```python
from build123d import *

# Parameters (mm, degrees)
F0_R     = 60
F1_DEPTH = 5
F3_DEPTH = 5.001
F4_R     = 58
F5_DEPTH = 3


with BuildPart() as f1:
    # F0 (on Top) → F1 (new body)
    with BuildSketch(Plane.XY):
        Circle(F0_R)
    extrude(amount=F1_DEPTH)

    # F2 (on face) → F3 (cut, through all)
    with BuildSketch(Plane.XY.offset(5)):
        with BuildLine():
            Line((-2.741307, 50.860289), (-2.800394, 53.905666))
            ThreePointArc((-2.800394, 53.905666), (-26.810197, 46.78331), (-44.999208, 29.568246))
            Line((-44.999208, 29.568246), (-42.39098, 27.998535))
            ThreePointArc((-42.39098, 27.998535), (-39.422273, 32.097611), (-36.032442, 35.855893))
            Line((-36.032442, 35.855893), (-31.764433, 31.624433))
            ThreePointArc((-31.764433, 31.624433), (-22.28061, 38.940283), (-11.190111, 43.46415))
            Line((-11.190111, 43.46415), (-12.704825, 49.321402))
            ThreePointArc((-12.704825, 49.321402), (-7.767263, 50.377001), (-2.741307, 50.860289))
        make_face()
        with BuildLine():
            Line((-53.808689, 0), (-44.738998, 0))
            ThreePointArc((-44.738998, 0), (-44.333174, 5.994104), (-43.11711, 11.877569))
            Line((-43.11711, 11.877569), (-48.95667, 13.487858))
            ThreePointArc((-48.95667, 13.487858), (-47.364057, 18.296418), (-45.259964, 22.904178))
            Line((-45.259964, 22.904178), (-47.967557, 24.430441))
            ThreePointArc((-47.967557, 24.430441), (-52.328709, 12.559654), (-53.808689, 0))
        make_face()
        with BuildLine():
            ThreePointArc((-43.11711, -11.832559), (-44.330124, -5.971391), (-44.738998, 0))
            Line((-44.738998, 0), (-53.808689, 0))
            ThreePointArc((-53.808689, 0), (-52.334607, -12.524554), (-47.995206, -24.365457))
            Line((-47.995206, -24.365457), (-45.342475, -22.814272))
            ThreePointArc((-45.342475, -22.814272), (-47.380636, -18.21008), (-48.948068, -13.42512))
            Line((-48.948068, -13.42512), (-43.11711, -11.832559))
        make_face()
        with BuildLine():
            Line((-42.377204, -28.020563), (-45.023724, -29.548192))
            ThreePointArc((-45.023724, -29.548192), (-26.781507, -46.767749), (-2.742129, -53.937126))
            Line((-2.742129, -53.937126), (-2.742129, -50.906584))
            ThreePointArc((-2.742129, -50.906584), (-7.777308, -50.376699), (-12.725699, -49.305607))
            Line((-12.725699, -49.305607), (-11.188747, -43.482557))
            ThreePointArc((-11.188747, -43.482557), (-22.268417, -38.947418), (-31.75433, -31.643718))
            Line((-31.75433, -31.643718), (-36.039297, -35.877891))
            ThreePointArc((-36.039297, -35.877891), (-39.414393, -32.115507), (-42.377204, -28.020563))
        make_face()
        with BuildLine():
            Line((0, -36.08707), (0, 0))
            Line((0, 0), (-17.828856, 0))
            ThreePointArc((-17.828856, 0), (-17.551636, -3.026807), (-16.733946, -5.954228))
            Line((-16.733946, -5.954228), (-33.773992, -11.896965))
            ThreePointArc((-33.773992, -11.896965), (-30.963522, -18.016735), (-27.060224, -23.504412))
            Line((-27.060224, -23.504412), (-13.459581, -11.657408))
            ThreePointArc((-13.459581, -11.657408), (-8.750525, -15.531259), (-3.038921, -17.66656))
            Line((-3.038921, -17.66656), (-6.482814, -35.405271))
            ThreePointArc((-6.482814, -35.405271), (-3.256267, -35.887467), (0, -36.08707))
        make_face()
        with BuildLine():
            Line((17.828856, 0), (0, 0))
            Line((0, 0), (0, -36.08707))
            ThreePointArc((0, -36.08707), (3.256267, -35.887467), (6.482814, -35.405271))
            Line((6.482814, -35.405271), (3.038921, -17.66656))
            ThreePointArc((3.038921, -17.66656), (8.750525, -15.531259), (13.459581, -11.657408))
            Line((13.459581, -11.657408), (27.060224, -23.504412))
            ThreePointArc((27.060224, -23.504412), (30.963522, -18.016735), (33.773992, -11.896965))
            Line((33.773992, -11.896965), (16.733946, -5.954228))
            ThreePointArc((16.733946, -5.954228), (17.551636, -3.026807), (17.828856, 0))
        make_face()
        with BuildLine():
            Line((0, 36.015704), (0, 0))
            Line((0, 0), (17.828856, 0))
            ThreePointArc((17.828856, 0), (17.554095, 3.040658), (16.733946, 5.981483))
            Line((16.733946, 5.981483), (33.78848, 11.882508))
            ThreePointArc((33.78848, 11.882508), (30.964356, 18.004289), (27.054407, 23.496481))
            Line((27.054407, 23.496481), (13.461306, 11.712858))
            ThreePointArc((13.461306, 11.712858), (8.780542, 15.595833), (3.079093, 17.712558))
            Line((3.079093, 17.712558), (6.480865, 35.418753))
            ThreePointArc((6.480865, 35.418753), (3.252606, 35.849388), (0, 36.015704))
        make_face()
        with BuildLine():
            Line((-17.828856, 0), (0, 0))
            Line((0, 0), (0, 36.015704))
            ThreePointArc((0, 36.015704), (-3.252606, 35.849388), (-6.480865, 35.418753))
            Line((-6.480865, 35.418753), (-3.079093, 17.712558))
            ThreePointArc((-3.079093, 17.712558), (-8.780542, 15.595833), (-13.461306, 11.712858))
            Line((-13.461306, 11.712858), (-27.054407, 23.496481))
            ThreePointArc((-27.054407, 23.496481), (-30.964356, 18.004289), (-33.78848, 11.882508))
            Line((-33.78848, 11.882508), (-16.733946, 5.981483))
            ThreePointArc((-16.733946, 5.981483), (-17.554095, 3.040658), (-17.828856, 0))
        make_face()
        with BuildLine():
            Line((2.742129, -50.906584), (2.742129, -53.937126))
            ThreePointArc((2.742129, -53.937126), (26.781507, -46.767749), (45.023724, -29.548192))
            Line((45.023724, -29.548192), (42.377204, -28.020563))
            ThreePointArc((42.377204, -28.020563), (39.414393, -32.115507), (36.039297, -35.877891))
            Line((36.039297, -35.877891), (31.75433, -31.643718))
            ThreePointArc((31.75433, -31.643718), (22.268417, -38.947418), (11.188747, -43.482557))
            Line((11.188747, -43.482557), (12.725699, -49.305607))
            ThreePointArc((12.725699, -49.305607), (7.777308, -50.376699), (2.742129, -50.906584))
        make_face()
        with BuildLine():
            ThreePointArc((43.11711, 11.877569), (44.333174, 5.994104), (44.738998, 0))
            Line((44.738998, 0), (53.808689, 0))
            ThreePointArc((53.808689, 0), (52.328709, 12.559654), (47.967557, 24.430441))
            Line((47.967557, 24.430441), (45.259964, 22.904178))
            ThreePointArc((45.259964, 22.904178), (47.364057, 18.296418), (48.95667, 13.487858))
            Line((48.95667, 13.487858), (43.11711, 11.877569))
        make_face()
        with BuildLine():
            Line((53.808689, 0), (44.738998, 0))
            ThreePointArc((44.738998, 0), (44.330124, -5.971391), (43.11711, -11.832559))
            Line((43.11711, -11.832559), (48.948068, -13.42512))
            ThreePointArc((48.948068, -13.42512), (47.380636, -18.21008), (45.342475, -22.814272))
            Line((45.342475, -22.814272), (47.995206, -24.365457))
            ThreePointArc((47.995206, -24.365457), (52.334607, -12.524554), (53.808689, 0))
        make_face()
        with BuildLine():
            Line((42.39098, 27.998535), (44.999208, 29.568246))
            ThreePointArc((44.999208, 29.568246), (26.810197, 46.78331), (2.800394, 53.905666))
            Line((2.800394, 53.905666), (2.741307, 50.860289))
            ThreePointArc((2.741307, 50.860289), (7.767263, 50.377001), (12.704825, 49.321402))
            Line((12.704825, 49.321402), (11.190111, 43.46415))
            ThreePointArc((11.190111, 43.46415), (22.28061, 38.940283), (31.764433, 31.624433))
            Line((31.764433, 31.624433), (36.032442, 35.855893))
            ThreePointArc((36.032442, 35.855893), (39.422273, 32.097611), (42.39098, 27.998535))
        make_face()
    extrude(amount=-F3_DEPTH, mode=Mode.SUBTRACT)

    # F4 (on face) → F5 (cut)
    with BuildSketch(Plane.XY.offset(5)):
        Circle(F4_R)
    extrude(amount=-F5_DEPTH, mode=Mode.SUBTRACT)


solid = f1.part
```
Design review of the part built by this model. Coordinates are the model's own, in mm. A direction names the side the tool comes from. Round coordinates to 2 decimals unless told otherwise and drop trailing zeros. Order: outer loops, then holes, each group sorted by start corner. A loop starts at its lowest first (then second) coordinate and runs counter-clockwise, first axis right, second up. Notation, with made-up numbers: (62.25, 24.25) - (96.25, 24.25) arc R9 cw to (96.25, 31.25) - close; hole circle Ø7 at (50, -27). An arc over 180 degrees is marked (long way). One line per question, with ' | ' between items.
Item 1: Take a section at C-C, the plane x = 25. Write out the cut boundary in (y, z), then the cut area to 3 significant figures.
Checks:
outline: (-54.54, 0) - (-47.75, 0) - (-47.75, 2) - (-52.34, 2) - (-52.34, 5) - (-54.54, 5) - close; (-37.24, 0) - (-21.71, 0) - (-21.71, 2) - (-37.24, 2) - close; (-8.84, 0) - (8.84, 0) - (8.84, 2) - (-8.84, 2) - close; (21.72, 0) - (37.24, 0) - (37.24, 2) - (21.72, 2) - close; (47.78, 0) - (54.54, 0) - (54.54, 5) - (52.34, 5) - (52.34, 2) - (47.78, 2) - close | area: 138 mm²
Item 2: For P1, Ø0.6, axis at y = -51.5, z = 1, coming from the -X side; P2, Ø3, axis at x = -6, y = -45.5, coming from the +Z side; P3, Ø1.6, axis at y = -52.5, z = 1, coming from the +X side, all flat-tipped, find the tip position at first contact; note any pin that passes through.
Checks:
P1: x = -31.28 | P2: z = 2 | P3: x = 30.45
Item 3: Wall thickness on line 1 (Y direction, x = -1.5, z = 4.15); line 2 (X direction, y = -1, z = 2.3); line 3 (X direction, y = 5, z = 0.9): over which ranges is each line inside the solid? List them lowest first. Write a range as [from, to].
Checks:
line 1: [-59.98, -57.98], [57.98, 59.98] | line 2: [-59.99, -57.99], [57.99, 59.99] | line 3: [-59.79, -53.58], [-44.46, -17.07], [17.07, 44.46], [53.58, 59.79]
Item 4: Draft analysis for pull direction X (two halves, no side actions). For faces 1 (the face through (-14.17, -12.49, 0)), 2 (the face through (30.916, -18.098, 1.014)), state which applies: +X half, -X half, draft (parallel to the pull), parting line (faces both ways), or undercut.
Checks:
face 1: draft | face 2: undercut
Item 5: Machinability: for faces 3 (the face through (-27.09, -46.59, 1.01)), 4 (the face through (-14, 14, 2)), which of the approach directions +Z, -Z, +X, -X, +Y, -Y give a long, thin tool a straight path to every point of the face, cutting with its end or side? Answer none if there is none.
Checks:
face 3: +Z, -Z | face 4: +Z
Item 6: Take a section at D-D, the plane z = 4. Write out the cut boundary in (x, y).
Checks:
outline: circle Ø120 at (0, 0); hole circle Ø116 at (0, 0)
Item 7: Take a section at B-B, the plane y = -45. Write out the cut boundary in (x, z), then the cut area to 3 significant figures.
Checks:
outline: (-39.69, 0) - (-29.64, 0) - (-29.64, 2) - (-36.59, 2) - (-36.59, 5) - (-39.69, 5) - close; (-11.59, 0) - (11.59, 0) - (11.59, 2) - (-11.59, 2) - close; (29.64, 0) - (39.69, 0) - (39.69, 5) - (36.59, 5) - (36.59, 2) - (29.64, 2) - close | area: 105 mm²
Item 8: Take a section at A-A, the plane x = -41. Write out the cut boundary in (y, z).
Checks:
outline: (-43.81, 0) - (-34.92, 0) - (-34.92, 2) - (-41.02, 2) - (-41.02, 5) - (-43.81, 5) - close; (-30.04, 0) - (30.03, 0) - (30.03, 2) - (-30.04, 2) - close; (34.94, 0) - (43.81, 0) - (43.81, 5) - (41.02, 5) - (41.02, 2) - (34.94, 2) - close
